Geometry check sheet. Reference: the model listing, model coordinates, mm. Face numbers are marked on the shaded views. A direction names the side the tool comes from. Give positions to 0.01 mm unless a question says otherwise; leave off trailing zeros. Loops run counter-clockwise (first coordinate to the right, second up) from the corner with the lowest first, then second, coordinate; pieces in that order, holes last.
```python
from build123d import *

# Parameters (mm, degrees)
SKETCH1_R           = 20.5
BOSS_EXTRUDE1_DEPTH = 15
SKETCH2_R           = 32.5
BOSS_EXTRUDE2_DEPTH = 7.5
SKETCH3_R           = 32
BOSS_EXTRUDE3_DEPTH = 7.5
SKETCH4_R           = 4
CUT_EXTRUDE1_DEPTH  = 30


with BuildPart() as part:
    # Sketch1 → Boss-Extrude1 (new body)
    with BuildSketch(Plane.XY):
        Circle(SKETCH1_R)
    extrude(amount=BOSS_EXTRUDE1_DEPTH)

    # Sketch2 → Boss-Extrude2 (add)
    with BuildSketch(Plane.XY.offset(15)):
        Circle(SKETCH2_R)
    extrude(amount=BOSS_EXTRUDE2_DEPTH)

    # Sketch3 → Boss-Extrude3 (add)
    with BuildSketch(Plane(origin=(0, 0, 0), x_dir=(-1, 0, 0), z_dir=(0, 0, -1))):
        Circle(SKETCH3_R)
    extrude(amount=BOSS_EXTRUDE3_DEPTH)

    # Sketch4 → Cut-Extrude1 (cut)
    with BuildSketch(Plane(origin=(0, 0, -7.5), x_dir=(-1, 0, 0), z_dir=(0, 0, -1))):
        Circle(SKETCH4_R)
    extrude(amount=-CUT_EXTRUDE1_DEPTH, mode=Mode.SUBTRACT)


solid = part.part
```
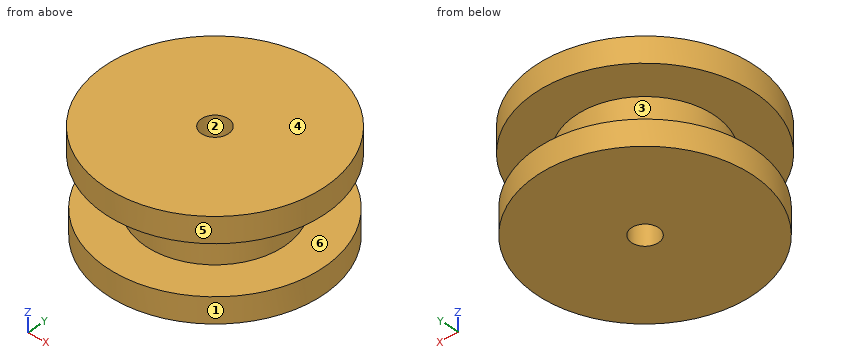
1) Tool access check on the marked faces 1, 2 and 3. Record the directions out of +Z, -Z, +X, -X, +Y, -Y that give a thin tool (end or side, any length) a straight path to the whole face; none if there is none.
2) Depth check by flat-ended pin: P1, Ø2, axis at y = -11.5, z = 0.5, coming from the +X side; P2, Ø3, axis at x = -19, z = 16, coming from the -Y side; P3, Ø6.5, axis at x = 0, y = 0, coming from the -Z side; P4, Ø10, axis at y = -26, z = 18, coming from the -X side. Enter the tip coordinate at first touch or a pass-through.
3) Sectioned sample at C-C on z = -3.5. Enter the section's corners in (x, y), plus the area to 3 significant figures.
4) Sectioned sample at D-D on y = -17. Enter the section's corners in (x, z), plus the area to 3 significant figures.
5) Sectioned sample at A-A on y = 0. Enter the section's corners in (x, z).
6) Scan lines: line 1 along Y through (x, z) = (0, 6.75); line 2 along Z through (x, y) = (-18.5, 22.5); line 3 along X through (y, z) = (-2.5, 5.75). Record each from-to range of solid material in increasing order.
7) Mould release check, pull along Z, two halves, no side actions. Record for the marked faces 4, 5 and 6: +Z half, -Z half, draft (parallel to the pull), parting line (faces both ways), or undercut.
Determined:
1. face 1: -Z
1. face 2: +Z, -Z
1. face 3: none
2. P1: stops at x = 30.18
2. P2: stops at y = -27.39
2. P3: passes through
2. P4: stops at x = -24.8
3. outline: circle Ø64 at (0, 0); hole circle Ø8 at (0, 0)
3. area: 3,170 mm2
4. outline: (-27.7, 15) - (-11.46, 15) - (-11.46, 0) - (-27.11, 0) - (-27.11, -7.5) - (27.11, -7.5) - (27.11, 0) - (11.46, 0) - (11.46, 15) - (27.7, 15) - (27.7, 22.5) - (-27.7, 22.5) - close
4. area: 1,170 mm2
5. outline: (-32.5, 15) - (-20.5, 15) - (-20.5, 0) - (-32, 0) - (-32, -7.5) - (-4, -7.5) - (-4, 22.5) - (-32.5, 22.5) - close; (4, -7.5) - (32, -7.5) - (32, 0) - (20.5, 0) - (20.5, 15) - (32.5, 15) - (32.5, 22.5) - (4, 22.5) - close
6. line 1: y = -20.5 to -4, 4 to 20.5
6. line 2: z = -7.5 to 0, 15 to 22.5
6. line 3: x = -20.35 to -3.12, 3.12 to 20.35
7. face 4: +Z half
7. face 5: draft
7. face 6: undercut
